```python
from build123d import *

# Parameters (mm, degrees)
SKETCH1_W           = 120
SKETCH1_H           = 120
BOSS_EXTRUDE1_DEPTH = 115
SKETCH2_W           = 110
SKETCH2_H           = 110
CUT_EXTRUDE1_DEPTH  = 110
SKETCH4_W           = 24
SKETCH4_H           = 30
CUT_EXTRUDE3_DEPTH  = 3
SKETCH6_R           = 7.75
CUT_EXTRUDE5_DEPTH  = 6
SKETCH9_W           = 30
SKETCH9_H           = 35
BOSS_EXTRUDE2_DEPTH = 3
FILLET2_R           = 2.5
SKETCH12_W          = 40
SKETCH12_H          = 50
CUT_EXTRUDE8_DEPTH  = 5
SKETCH13_W          = 50
SKETCH13_H          = 60
CUT_EXTRUDE9_DEPTH  = 3
SKETCH14_W          = 40
SKETCH14_H          = 60
CUT_EXTRUDE10_DEPTH = 3


with BuildPart() as part:
    # Sketch1 → Boss-Extrude1 (new body)
    with BuildSketch(Plane(origin=(0, 0, 0), x_dir=(1, 0, 0), z_dir=(0, 1, 0))):
        with Locations((0.113396959, 0)):
            Rectangle(SKETCH1_W, SKETCH1_H)
    extrude(amount=BOSS_EXTRUDE1_DEPTH)

    # Sketch2 → Cut-Extrude1 (cut)
    with BuildSketch(Plane.XZ):
        with Locations((0.113396959, 0)):
            Rectangle(SKETCH2_W, SKETCH2_H)
    extrude(amount=-CUT_EXTRUDE1_DEPTH, mode=Mode.SUBTRACT)

    # Sketch4 → Cut-Extrude3 (cut)
    with BuildSketch(Plane(origin=(60.113396959, 0, 0), x_dir=(0, 0, -1), z_dir=(1, 0, 0))):
        with Locations((0, 100)):
            Rectangle(SKETCH4_W, SKETCH4_H)
    extrude(amount=-CUT_EXTRUDE3_DEPTH, mode=Mode.SUBTRACT)

    # Sketch6 → Cut-Extrude5 (cut)
    with BuildSketch(Plane(origin=(0, 0, -60), x_dir=(-1, 0, 0), z_dir=(0, 0, -1))):
        with Locations((-35.113396959, 90)):
            Circle(SKETCH6_R)
    extrude(amount=-CUT_EXTRUDE5_DEPTH, mode=Mode.SUBTRACT)

    # Sketch9 → Boss-Extrude2 (add)
    with BuildSketch(Plane.ZY.offset(-55.113396959)):
        with Locations((0, 92.5)):
            Rectangle(SKETCH9_W, SKETCH9_H)
    extrude(amount=BOSS_EXTRUDE2_DEPTH)

    # Fillet2
    fillet2_edges = [part.edges().sort_by_distance(p)[0] for p in [
        (60.113396959, 115, 36),
        (0.113396959, 115, -60),
        (60.113396959, 115, -36),
        (-59.886603041, 115, 0),
        (0.113396959, 115, 60),
        (-59.886603041, 57.5, -60),
        (60.113396959, 57.5, -60),
        (60.113396959, 57.5, 60),
        (-59.886603041, 57.5, 60),
    ]]
    fillet(fillet2_edges, radius=FILLET2_R)

    # Sketch12 → Cut-Extrude8 (cut)
    with BuildSketch(Plane.ZY.offset(59.886603041)):
        with Locations((20, 75)):
            Rectangle(SKETCH12_W, SKETCH12_H)
    extrude(amount=-CUT_EXTRUDE8_DEPTH, mode=Mode.SUBTRACT)

    # Sketch13 → Cut-Extrude9 (cut)
    with BuildSketch(Plane.ZY.offset(59.886603041)):
        with Locations((20, 75)):
            Rectangle(SKETCH13_W, SKETCH13_H)
    extrude(amount=-CUT_EXTRUDE9_DEPTH, mode=Mode.SUBTRACT)

    # Sketch14 → Cut-Extrude10 (cut)
    with BuildSketch(Plane.ZY.offset(59.886603041)):
        with Locations((-30, 75)):
            Rectangle(SKETCH14_W, SKETCH14_H)
    extrude(amount=-CUT_EXTRUDE10_DEPTH, mode=Mode.SUBTRACT)


solid = part.part
```
The listing builds one solid part. Answer for the finished solid, in the listing's coordinates (mm). A direction names the side the tool comes from. Round coordinates to 2 decimals unless told otherwise and drop trailing zeros. Order: outer loops, then holes, each group sorted by start corner. A loop starts at its lowest first (then second) coordinate and runs counter-clockwise, first axis right, second up. Notation, with made-up numbers: (-22, 74) - (20, 74) arc R31 cw to (20, 113) - close; hole circle Ø11 at (74, -37). An arc over 180 degrees is marked (long way). Put each result on its own line as item: value. Start each with the question number.
(1) Find section B-B (y = 42). Give the vertices of the cut face in (x, z), plus the area to 3 significant figures.
(2) Given P1, Ø3, axis at x = -38, z = -32.5, coming from the -Y side; P2, Ø1.5, axis at x = -59, y = 75.5, coming from the -Z side; P3, Ø2.5, axis at x = -59, y = 71, coming from the +Z side, each flat-ended and moving along its own axis, determine where each tip first touches the part or whether it passes through.
(3) Determine the mould class of faces 6 (the flat face through (52.113, 93, 0)), 7 (the flat face through (60.113, 55, 1)), 8 (the flat face through (-1, 55, -60)) for opening direction Z: released by +Z, released by -Z, zero draft, split by the parting line, or undercut.
(4) Find section A-A (z = 20). Give the vertices of the cut face in (x, y).
(5) Find section D-D (z = -26.5). Give the vertices of the cut face in (x, y).
(6) Straight lines are drawn through the part: probe 1 along Z at (x, y) = (-1, 58); probe 2 along X at (y, z) = (64.5, -38); probe 3 along X at (y, z) = (98, -1.5). For each, find the intervals that lie inside material, in ascending order. Write a range as from..to.
(7) For faces 1 (the flat face through (57.113, 100, 0)), 2 (the flat face through (-56.887, 75, 42)), 3 (the flat face through (-1, 54, -55)), 4 (the flat face through (-5, 0, 57)), 5 (the cylindrical face through (41.26, 85.28, -57.54)), determine the directions among +Z, -Z, +X, -X, +Y, -Y from which every point of the face is accessible in a straight line to the end or side of a thin tool.
(8) Find section C-C (x = 12). Give the vertices of the cut face in (y, z).
Reply:
1. outline: (-59.89, -57.5) arc R2.5 ccw to (-57.39, -60) - (57.61, -60) arc R2.5 ccw to (60.11, -57.5) - (60.11, 57.5) arc R2.5 ccw to (57.61, 60) - (-57.39, 60) arc R2.5 ccw to (-59.89, 57.5) - close; hole (-54.89, -55) - (55.11, -55) - (55.11, 55) - (-54.89, 55) - close
1. area: 2,290 mm^2
2. P1: y = 110
2. P2: z = -59.85
2. P3: z = 59.97
3. face 6: undercut
3. face 7: zero draft
3. face 8: released by -Z
4. outline: (-59.89, 0) - (-54.89, 0) - (-54.89, 50) - (-56.89, 50) - (-56.89, 45) - (-59.89, 45) - close; (-59.89, 105) - (-56.89, 105) - (-56.89, 100) - (-54.89, 100) - (-54.89, 110) - (55.11, 110) - (55.11, 0) - (60.11, 0) - (60.11, 112.5) arc R2.5 ccw to (57.61, 115) - (-57.39, 115) arc R2.5 ccw to (-59.89, 112.5) - close
5. outline: (-59.89, 0) - (-54.89, 0) - (-54.89, 110) - (55.11, 110) - (55.11, 0) - (60.11, 0) - (60.11, 112.5) arc R2.5 ccw to (57.61, 115) - (-57.39, 115) arc R2.5 ccw to (-59.89, 112.5) - (-59.89, 105) - (-56.89, 105) - (-56.89, 45) - (-59.89, 45) - close
6. probe 1: -60..-55, 55..60
6. probe 2: -56.89..-54.89, 55.11..60.11
6. probe 3: -56.89..-54.89, 52.11..57.11
7. face 1: +X, +Y
7. face 2: -X
7. face 3: -Y
7. face 4: +Z, -Z, +X, -X, -Y
7. face 5: -Z
8. outline: (0, -60) - (112.5, -60) arc R2.5 ccw to (115, -57.5) - (115, 57.5) arc R2.5 ccw to (112.5, 60) - (0, 60) - (0, 55) - (110, 55) - (110, -55) - (0, -55) - close
